Job drawing, mm, ordinate dimensions from the low corner. One solid piece. Round coordinates to 2 decimals unless told otherwise and drop trailing zeros. Order: outer loops, then holes, each group sorted by start corner. A loop starts at its lowest first (then second) coordinate and runs counter-clockwise, first axis right, second up. Notation, with made-up numbers: (74.25, 10.25) -> (130.25, 10.25) arc R12 cw to (130.25, 33.25) -> close; hole circle Ø5 at (-38.75, 80). An arc over 180 degrees is marked (long way). Return JSON: item names as keys, results as strings. Group by question number.
Q1. Cut at B-B (z = 6.5). Write the cut outline in (x, y).
Q2. Cut at A-A (x = 6.5). Write the cut outline in (y, z).
Q3. Cut at D-D (x = 12). Write the cut outline in (y, z).
Q4. Mould opens along Z. For the marked faces 1, 2 and 3 say: +Z half, -Z half, draft (parallel to the pull), parting line (faces both ways), or undercut.
Q5. Probe line 1 along Y through (x, z) = (3, 1.25); line 2 along Z through (x, y) = (6.5, 6); line 3 along Z through (x, y) = (6.5, 9.25). List the from-to ranges inside material, lowest first.
Q6. Cut at C-C (y = 1.25). Write the cut outline in (x, z).
Q7. Flat gauge pins, fed straight in: pin 1 (6 mm diameter, centred on x = 6.5, z = 6.5, fed in from -Y); pin 2 (2 mm diameter, centred on x = 9.5, y = 7, fed in from +Z) (1 decimal). Where does each tip first touch, or does it go through?
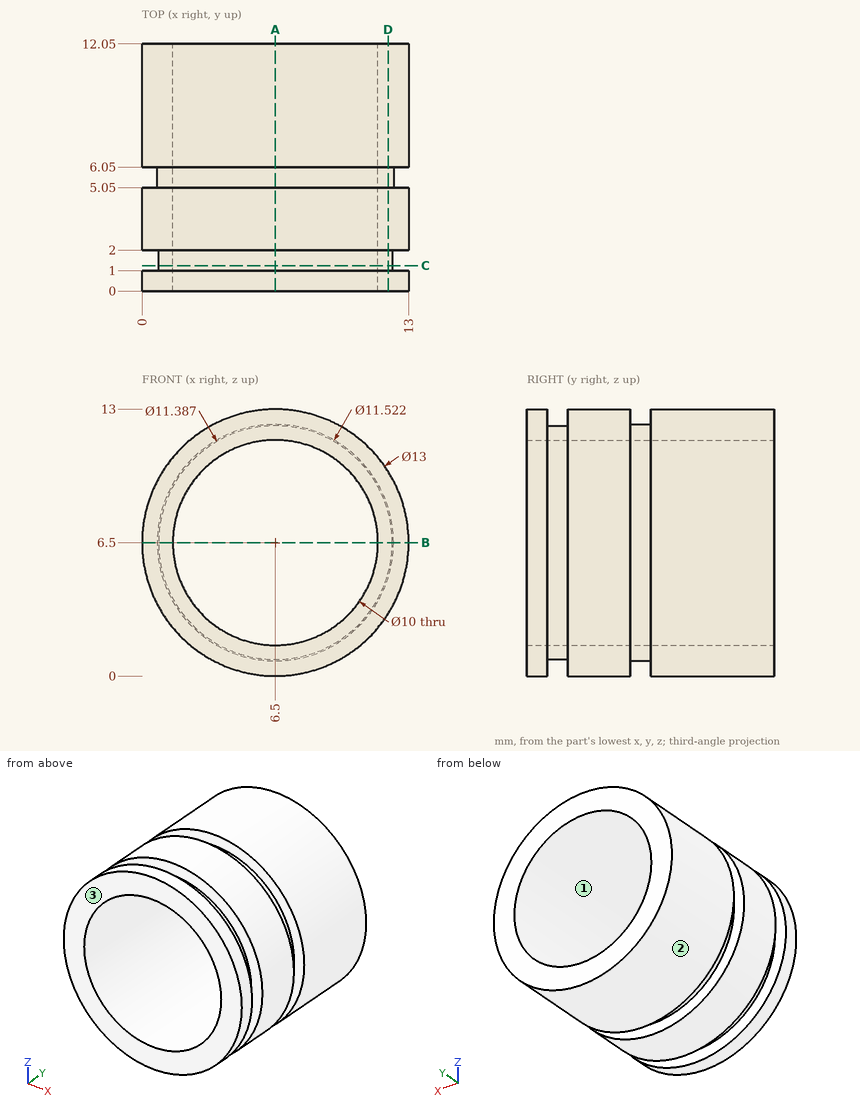
Solution:
{
 "1": {"outline": "(0, 0) -> (1.5, 0) -> (1.5, 12.05) -> (0, 12.05) -> (0, 6.05) -> (0.74, 6.05) -> (0.74, 5.05) -> (0, 5.05) -> (0, 2) -> (0.81, 2) -> (0.81, 1) -> (0, 1) -> close; (11.5, 0) -> (13, 0) -> (13, 1) -> (12.19, 1) -> (12.19, 2) -> (13, 2) -> (13, 5.05) -> (12.26, 5.05) -> (12.26, 6.05) -> (13, 6.05) -> (13, 12.05) -> (11.5, 12.05) -> close"},
 "2": {"outline": "(0, 0) -> (1, 0) -> (1, 0.81) -> (2, 0.81) -> (2, 0) -> (5.05, 0) -> (5.05, 0.74) -> (6.05, 0.74) -> (6.05, 0) -> (12.05, 0) -> (12.05, 1.5) -> (0, 1.5) -> close; (0, 11.5) -> (12.05, 11.5) -> (12.05, 13) -> (6.05, 13) -> (6.05, 12.26) -> (5.05, 12.26) -> (5.05, 13) -> (2, 13) -> (2, 12.19) -> (1, 12.19) -> (1, 13) -> (0, 13) -> close"},
 "3": {"outline": "(0, 3.04) -> (1, 3.04) -> (1, 5.03) -> (2, 5.03) -> (2, 3.04) -> (5.05, 3.04) -> (5.05, 4.79) -> (6.05, 4.79) -> (6.05, 3.04) -> (12.05, 3.04) -> (12.05, 9.96) -> (6.05, 9.96) -> (6.05, 8.21) -> (5.05, 8.21) -> (5.05, 9.96) -> (2, 9.96) -> (2, 7.97) -> (1, 7.97) -> (1, 9.96) -> (0, 9.96) -> close"},
 "4": {"face 1": "undercut", "face 2": "parting line", "face 3": "draft"},
 "5": {"line 1": "y = 0 to 1, 2 to 5.05, 6.05 to 12.05", "line 2": "z = 0.74 to 1.5, 11.5 to 12.26", "line 3": "z = 0 to 1.5, 11.5 to 13"},
 "6": {"outline": "circle Ø11.39 at (6.5, 6.5); hole circle Ø10 at (6.5, 6.5)"},
 "7": {"pin 1": "passes through", "pin 2": "stops at z = 12.7"}
}
